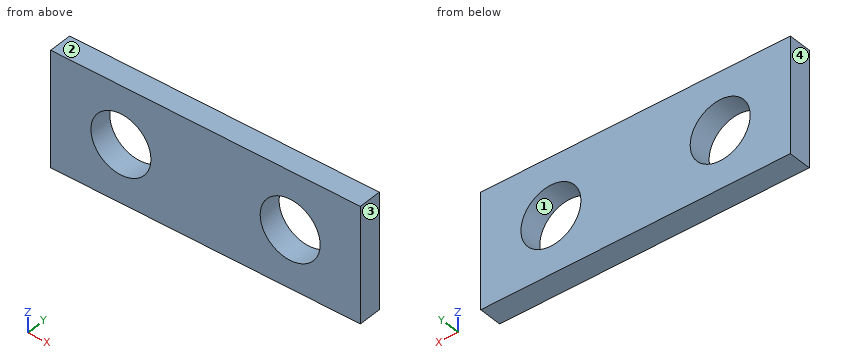
from build123d import *

# Parameters (mm, degrees)
SKETCH1_W           = 40.25
SKETCH1_H           = 15
BOSS_EXTRUDE1_DEPTH = 3
CUT_EXTRUDE1_START  = -4
SKETCH2_R           = 3.9
CUT_EXTRUDE1_DEPTH  = 5


with BuildPart() as part:
    # Sketch1 → Boss-Extrude1 (new body)
    with BuildSketch(Plane(origin=(0, 0, 0), x_dir=(1, 0, 0), z_dir=(0, 1, 0))):
        Rectangle(SKETCH1_W, SKETCH1_H)
    extrude(amount=BOSS_EXTRUDE1_DEPTH)

    # Sketch2 → Cut-Extrude1 (cut)
    with BuildSketch(Plane(origin=(0, 3, 0), x_dir=(1, 0, 0), z_dir=(0, 1, 0)).offset(CUT_EXTRUDE1_START)):
        with Locations((-11, 0)):
            Circle(SKETCH2_R)
    cut_extrude1 = extrude(amount=CUT_EXTRUDE1_DEPTH, mode=Mode.SUBTRACT)

    # Mirror1: Cut-Extrude1 across plane
    add(cut_extrude1.mirror(Plane(origin=(0, 0, 0), x_dir=(0, 0, 1), z_dir=(1, 0, 0))), mode=Mode.SUBTRACT)


solid = part.part
Could you check a few things on this model? Use its own coordinates, in mm. Face numbers are marked on the shaded views. Give positions to 0.01 mm unless a question says otherwise; leave off trailing zeros. Loops run counter-clockwise (first coordinate to the right, second up) from the corner with the lowest first, then second, coordinate; pieces in that order, holes last. Notation, with made-up numbers: M 27.25,84.5 L 37.25,84.5 A25 cw 37.25,102.5 Z; hole C 41.25,-33 d2. An arc over 180 degrees is marked long. Answer as a JSON object with one key per item and string values.
Q1. Suppose I cut it at C-C, the plane y = 0.6. List the corners of the cut face in (x, z) for me (3 decimals).
Values found:
{"outline": "M -20.125,-7.5 L 20.125,-7.5 L 20.125,7.5 L -20.125,7.5 Z; hole C -11,0 d7.8; hole C 11,0 d7.8"}
Q2. If we mould it in two halves opening along X, with no side actions, what happens to the marked faces 1, 2, 3 and 4? For each: pulls with the +X half, pulls with the -X half, needs draft (parallel to the pull), parting line crosses it, or undercut.
Values found:
{"face 1": "undercut", "face 2": "needs draft", "face 3": "pulls with the +X half", "face 4": "pulls with the -X half"}
Q3. Suppose I cut it at B-B, the plane x = 8.5. List the corners of the cut face in (y, z) for me.
Values found:
{"outline": "M 0,-7.5 L 3,-7.5 L 3,-2.99 L 0,-2.99 Z; M 0,2.99 L 3,2.99 L 3,7.5 L 0,7.5 Z"}
Q4. Suppose I cut it at D-D, the plane z = 2.5. List the corners of the cut face in (x, y) for me (3 decimals).
Values found:
{"outline": "M -20.125,0 L -13.993,0 L -13.993,3 L -20.125,3 Z; M -8.007,0 L 8.007,0 L 8.007,3 L -8.007,3 Z; M 13.993,0 L 20.125,0 L 20.125,3 L 13.993,3 Z"}
Q5. For P1, Ø6, axis at x = -11, z = 0, coming from the -Y side, with a flat end and sliding along its axis, tell me the tip position at first contact or that it passes through.
Values found:
{"P1": "passes through"}
Q6. Suppose I cut it at A-A, the plane z = 0. List the corners of the cut face in (x, y) for me (3 decimals), plus the area to 4 significant figures.
Values found:
{"outline": "M -20.125,0 L -14.9,0 L -14.9,3 L -20.125,3 Z; M -7.1,0 L 7.1,0 L 7.1,3 L -7.1,3 Z; M 14.9,0 L 20.125,0 L 20.125,3 L 14.9,3 Z", "area": "73.95 mm²"}
Q7. If I drill on probe 1 along Z at (x, y) = (11, 2.2); probe 2 along X at (y, z) = (1.4, 3.5) (3 decimals); probe 3 along Z at (x, y) = (10, 1.8), over which ranges is the centre line in solid material (lowest first)? Write a range as [from, to].
Values found:
{"probe 1": "z = [-7.5, -3.9], [3.9, 7.5]", "probe 2": "x = [-20.125, -12.72], [-9.28, 9.28], [12.72, 20.125]", "probe 3": "z = [-7.5, -3.77], [3.77, 7.5]"}
